Autodesk Fusion 360 part; units mm, degrees
sketch "Sketch1" plane through (0, 0, 0) normal (0, 0, 1) x (1, 0, 0) in component "Component"
  line L0 (80, -100) -> (-80, -100)
  line L1 (-80, -100) -> (-80, 100)
  line L2 (-80, 100) -> (80, 100)
  line L3 (80, 100) -> (80, -100)
  line L4 (80, -100) -> (-80, 100) construction
  line L5 (-80, -100) -> (80, 100) construction
  dimension "d1" = 160
  dimension "d2" = 200
extrude "Extrude1" add sketch "Sketch1" along normal blind 60 in component "Component"
sketch "Sketch5" plane through (0, 0, 60) normal (0, 0, 1) x (-1, 0, 0) in component "Component"
  line L0 (-80, -100) -> (80, -100)
  line L1 (80, -100) -> (80, 100)
  line L2 (80, 100) -> (-80, 100)
  line L3 (-80, 100) -> (-80, -100)
  line L4 (-20, 100) -> (-80, 40)
extrude "Extrude3" cut sketch "Sketch5" against normal up to surface (60 mm away) contours L2 L3 L4 in component "Component"
sketch "Sketch6" plane through (0, 0, 60) normal (0, 0, 1) x (-1, 0, 0) in component "Component"
  line L0 (-20, 100) -> (-80, 40)
  line L1 (-80, 40) -> (-80, -100)
  line L2 (-80, -100) -> (80, -100)
  line L3 (80, -100) -> (80, 100)
  line L4 (80, 100) -> (-20, 100)
  line L5 (60, 100) -> (60, 60)
  line L6 (60, 60) -> (0, 0)
  line L7 (0, 0) -> (0, -60)
  line L8 (0, -60) -> (80, -60)
  line L9 (80, 100) -> (60, 100)
extrude "Extrude4" add sketch "Sketch6" along normal blind 40 contours L3 L4 L5 L6 L7 L8 L9 in component "Component"
sketch "Sketch7" plane through (0, 0, 60) normal (0, 0, 1) x (-1, 0, 0) in component "Component"
  line L0 (60, 60) -> (60, 100)
  line L1 (60, 100) -> (-20, 100)
  line L2 (-20, 100) -> (-80, 40)
  line L3 (-80, 40) -> (-80, -100)
  line L4 (-80, -100) -> (80, -100)
  line L5 (80, -100) -> (80, -60)
  line L6 (80, -60) -> (0, -60)
  line L7 (0, -60) -> (0, 0)
  line L8 (0, 0) -> (60, 60)
  line L9 (-60, -60) -> (-80, -80)
  line L10 (-80, -100) -> (80, -100)
  line L11 (80, -60) -> (-60, -60)
extrude "Extrude5" add sketch "Sketch7" along normal blind 60 contours L3 L4 L5 L6 L9 L10 L11 in component "Component"
sketch "Sketch8" plane through (0, 0, 100) normal (0, 0, 1) x (-1, 0, 0) in component "Component"
  line L0 (80, 100) -> (60, 100)
  line L1 (60, 100) -> (60, 60)
  line L2 (60, 60) -> (0, 0)
  line L3 (0, 0) -> (0, -60)
  line L4 (0, -60) -> (80, -60)
  line L5 (80, -60) -> (80, 100)
  circle A0 centre (40, -30) radius 10
  dimension "d14" = 40
  dimension "d15" = 30
  dimension "d16" = 20
extrude "Extrude6" cut sketch "Sketch8" against normal up to surface (100 mm away) contours A0 in component "Component"
sketch "Sketch9" plane through (0, 60, 0) normal (0, -1, 0) x (1, 0, 0) in component "Component"
  line L0 (-80, 100) -> (0, 100)
  line L1 (0, 100) -> (0, 60)
  line L2 (0, 60) -> (60, 60)
  line L3 (60, 60) -> (60, 120)
  line L4 (60, 120) -> (-80, 120)
  line L5 (-80, 120) -> (-80, 100)
  circle A0 centre (30, 90) radius 10
  dimension "d19" = 30
  dimension "d20" = 30
  dimension "d21" = 20
extrude "Extrude7" cut sketch "Sketch9" against normal up to surface (40 mm away) contours A0 in component "Component"
component "Component" placed x (1, 0, 0) y (0, 1, 0) z (0, 0, 1) at (0, 0, 0)
Part model, mm, in its own coordinate system. A direction names the side the tool comes from. Round coordinates to 2 decimals unless told otherwise and drop trailing zeros. Loops run counter-clockwise (first coordinate to the right, second up) from the corner with the lowest first, then second, coordinate; pieces in that order, holes last.
1. Slice it at C-C (x = 30). Give the cut face in (y, z).
Solutions:
outline: (-90, 0) - (100, 0) - (100, 80) - (60, 80) - (60, 60) - (-90, 60) - close; (60, 100) - (100, 100) - (100, 120) - (60, 120) - close
2. Drill centre lines: line 1 along Z through (x, y) = (30, 88); line 2 along X through (y, z) = (30, 72.5); line 3 along X through (y, z) = (30, 24.5). Where is each one in solid material? Low to high.
Solutions:
line 1: z = 0 to 80, 100 to 120
line 2: x = -80 to -50, -30 to 0
line 3: x = -80 to -50, -30 to 80
3. Slice it at A-A (z = 90). Give the cut face in (x, y).
Solutions:
outline: (-80, -100) - (-60, -100) - (-60, -60) - (0, 0) - (0, 60) - (20, 60) - (20, 100) - (-80, 100) - close; (40, 60) - (60, 60) - (80, 80) - (80, 100) - (40, 100) - close; hole circle Ø20 at (-40, 30)
4. Slice it at D-D (z = 47). Give the cut face in (x, y).
Solutions:
outline: (-80, -100) - (20, -100) - (80, -40) - (80, 100) - (-80, 100) - close; hole circle Ø20 at (-40, 30)
5. 3-axis set-ups, long thin cutter, end or side, ignore diameter. For faces 1 (the face through (-48, -3, 100)), 2 (the face through (-30, -30, 80)), 3 (the face through (50, -70, 30)): which of +Z, -Z, +X, -X, +Y, -Y reach the whole face in a straight line?
Solutions:
face 1: +Z, +X, -X, -Y
face 2: +Z, +X, -Y
face 3: +Z, -Z, +X, -Y
6. Two-plate mould, pull along Y, no slides. Class faces 4 (the face through (70, 70, 90)), 5 (the face through (-37.83, 39.76, 50.7)), 6 (the face through (-60, -80, 80)): pulls with the +Y half, pulls with the -Y half, needs draft (parallel to the pull), parting line crosses it, or undercut.
Solutions:
face 4: pulls with the -Y half
face 5: undercut
face 6: needs draft
7. Flat gauge pin, fed straight in: pin 1 (12 mm diameter, centred on x = 30, z = 90, fed in from +Y) (1 decimal). Where does the tip first touch, or does it go through?
Solutions:
pin 1: passes through
8. Slice it at B-B (y = 30). Give the cut face in (x, z), and give its area (3 significant figures).
Solutions:
outline: (-80, 0) - (-50, 0) - (-50, 100) - (-80, 100) - close; (-30, 0) - (80, 0) - (80, 60) - (0, 60) - (0, 100) - (-30, 100) - close
area: 10,800 mm2
